Geometry: final body of the model. Coordinates: model frame, mm. Face numbers are marked on the shaded views. Coordinates: 2 decimals unless noted, no trailing zeros. Loops run counter-clockwise (first coordinate to the right, second up) from the corner with the lowest first, then second, coordinate; pieces in that order, holes last. Notation, with made-up numbers: (80.25, 89) - (119.25, 89) arc R30 cw to (119.25, 123) - close; hole circle Ø5 at (27.5, 24.25). An arc over 180 degrees is marked (long way). Put each result on its own line as item: value. Start each with the question number.
1) Section C-C on x = 14. Output: boundary loops of the cut face in (y, z) (3 decimals).
2) Draft query along X for the marked faces 1, 2 and 3. Return one class per face: +X half, -X half, draft (parallel to the pull), parting line (faces both ways), or undercut.
3) Section A-A on y = 10. Output: boundary loops of the cut face in (x, z) (3 decimals).
4) Section B-B on x = 0. Output: boundary loops of the cut face in (y, z) (3 decimals).
5) Material intervals for line 1 along Z through (x, y) = (-12.5, 4) (3 decimals); line 2 along Y through (x, z) = (0, -2.6); line 3 along Z through (x, y) = (-2.5, -3.5) (3 decimals), sorted ascending. Write a range as from..to.
6) Contact query for flat-ended pins moving along their axis: pin 1 Ø5 at (y, z) = (0.5, 28.5) entering from -X; pin 2 Ø8 at (y, z) = (8, 19) entering from -X; pin 3 Ø3 at (x, z) = (2, 32.5) entering from -Y; pin 4 Ø13.5 at (x, y) = (5, -6) entering from +Z. Output: stop coordinate, or through.
```python
from build123d import *

# Parameters (mm, degrees)
F0_R     = 22.86
F1_DEPTH = 5.334
F2_R     = 8.763
F3_DEPTH = 38.1
F3_TAPER = 2.5
F4_T     = -2.159


with BuildPart() as f1:
    # F0 (on Top) → F1 (new body)
    with BuildSketch(Plane.XY):
        Circle(F0_R)
    extrude(amount=-F1_DEPTH)

    # F2 (on Top) → F3 (join)
    with BuildSketch(Plane.XY):
        Circle(F2_R)
    extrude(amount=F3_DEPTH, taper=F3_TAPER)

    # F4
    f4_openings = [f1.faces().sort_by_distance(p)[0] for p in [
        (0, 0, 38.1),
    ]]
    offset(amount=F4_T, openings=f4_openings, kind=Kind.INTERSECTION)


solid = f1.part
```
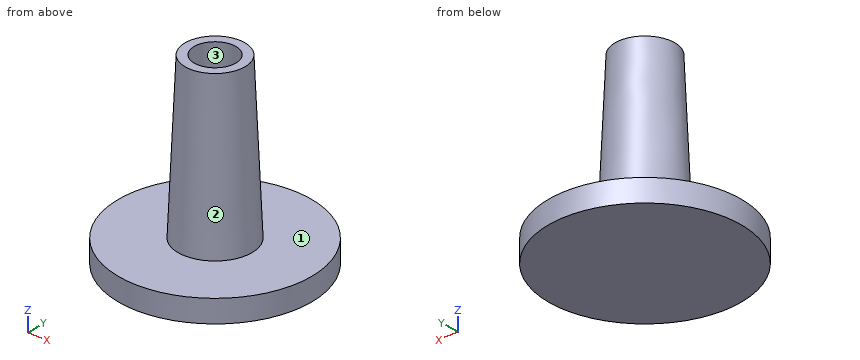
Answer block:
1. outline: (-18.072, -5.334) - (18.072, -5.334) - (18.072, 0) - (-18.072, 0) - close; hole (-15.249, -3.175) - (15.249, -3.175) - (15.249, -2.159) - (-15.249, -2.159) - close
2. face 1: draft
2. face 2: parting line
2. face 3: undercut
3. outline: (-20.557, -5.334) - (20.557, -5.334) - (20.557, 0) - (-20.557, 0) - close; hole (-18.125, -3.175) - (18.125, -3.175) - (18.125, -2.159) - (-18.125, -2.159) - close
4. outline: (-22.86, -5.334) - (22.86, -5.334) - (22.86, 0) - (8.763, 0) - (7.1, 38.1) - (4.938, 38.1) - (6.696, -2.159) - (20.701, -2.159) - (20.701, -3.175) - (-20.701, -3.175) - (-20.701, -2.159) - (-6.696, -2.159) - (-4.938, 38.1) - (-7.1, 38.1) - (-8.763, 0) - (-22.86, 0) - close
5. line 1: z = -5.334..-3.175, -2.159..0
5. line 2: y = -22.86..-20.7, 20.7..22.86
5. line 3: z = -5.334..-3.175
6. pin 1: stops at x = -7.63
6. pin 2: stops at x = -6.86
6. pin 3: stops at y = -7.34
6. pin 4: stops at z = 38.1
